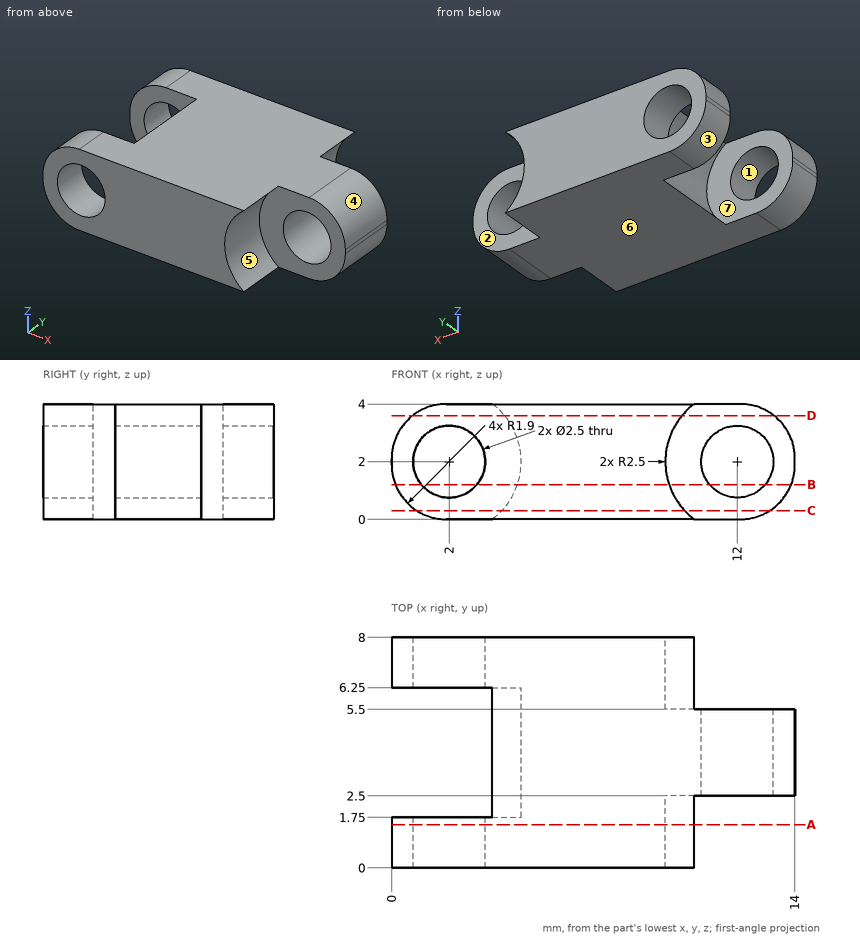
Study the drawing (mm; zero at the part's minimum x, y, z) and answer. A direction names the side the tool comes from. Round coordinates to 2 decimals unless told otherwise and drop trailing zeros. Write each loop counter-clockwise with the first axis right and the second up, starting at its lowest first coordinate (ties: lowest second). Pieces come first, ordered by that corner, then holes.
1) A cutting plane is placed at A-A on y = 1.5. Determine the outline of the cut face in (x, z).
2) A cutting plane is placed at D-D on z = 3.6. Determine the outline of the cut face in (x, y), and give its area (3 significant figures).
3) Flat-ended cylindrical pins translate along their axes: P1, Ø2, axis at y = 3.5, z = 3.5, coming from the +X side; P2, Ø1, axis at y = 4.5, z = 3, coming from the -X side; P3, Ø1.5, axis at x = 12, z = 2, coming from the -Y side; P4, Ø1.2, axis at x = 11, z = 2, coming from the +Y side. Find the tip coordinate at first contact, or state that the pin passes through.
4) Which of the six approach directions +Z, -Z, +X, -X, +Y, -Y give full straight-line access (tool end or side, diameter ignored) to the marked faces 5, 6 and 7?
5) A cutting plane is placed at C-C on z = 0.3. Determine the outline of the cut face in (x, y).
6) Determine the mould class of the marked faces 1, 2, 3 and 4 for opening direction Z: pulls with the +Z half, pulls with the -Z half, needs draft (parallel to the pull), parting line crosses it, or undercut.
7) Consider probe 1 along Z at (x, y) = (2, 1.2); probe 2 along Y at (x, z) = (4.25, 1.15); probe 3 along X at (y, z) = (0.5, 2.35). Determine where each line is inside the solid, lowest interval first.
8) A cutting plane is placed at B-B on z = 1.2. Determine the outline of the cut face in (x, y).
Entries:
1. outline: (0, 1.9) arc R1.9 ccw to (1.9, 0) - (10.5, 0) arc R2.5 cw to (10.5, 4) - (1.9, 4) arc R1.9 ccw to (0, 2.1) - close; hole circle Ø2.5 at (2, 2)
2. outline: (0.73, 0) - (10.08, 0) - (10.08, 2.5) - (13.27, 2.5) - (13.27, 5.5) - (10.08, 5.5) - (10.08, 8) - (0.73, 8) - (0.73, 6.25) - (3.92, 6.25) - (3.92, 1.75) - (0.73, 1.75) - close
2. area: 70.0 mm2
3. P1: stops at x = 13.96
3. P2: stops at x = 4
3. P3: passes through
3. P4: stops at y = 5.5
4. face 5: +X, -Y
4. face 6: -Z, +X, -X, +Y, -Y
4. face 7: -X
5. outline: (0.88, 0) - (10.17, 0) - (10.17, 2.5) - (13.12, 2.5) - (13.12, 5.5) - (10.17, 5.5) - (10.17, 8) - (0.88, 8) - (0.88, 6.25) - (3.83, 6.25) - (3.83, 1.75) - (0.88, 1.75) - close
6. face 1: undercut
6. face 2: undercut
6. face 3: pulls with the -Z half
6. face 4: pulls with the +Z half
7. probe 1: z = 0 to 0.75, 3.25 to 4
7. probe 2: y = 0 to 1.75, 6.25 to 8
7. probe 3: x = 0.02 to 0.8, 3.2 to 9.52
8. outline: (0.13, 0) - (1.04, 0) - (1.04, 1.75) - (0.13, 1.75) - close; (0.13, 6.25) - (1.04, 6.25) - (1.04, 8) - (0.13, 8) - close; (2.96, 0) - (9.63, 0) - (9.63, 2.5) - (11.04, 2.5) - (11.04, 5.5) - (9.63, 5.5) - (9.63, 8) - (2.96, 8) - (2.96, 6.25) - (4.37, 6.25) - (4.37, 1.75) - (2.96, 1.75) - close; (12.96, 2.5) - (13.87, 2.5) - (13.87, 5.5) - (12.96, 5.5) - close
